```python
from build123d import *

# Parameters (mm, degrees)
SKICA1_R                  = 30
SKICA1_R_2                = 15
P_IDAT_VYSUNUT_M1_DEPTH   = 80
ZKOSEN_1_SIZE             = 1
M8_Z_VIT1_REACH           = 62
M8_Z_VIT1_BORE_R          = 3.4
M8_Z_VIT1_ON_FACE_2_REACH = 72.981
M8_Z_VIT1_BORE_2_R        = 3.4
M8_Z_VIT2_REACH           = 62
M8_Z_VIT2_BORE_R          = 3.4
KRUHOV_POLE1_COUNT        = 2
KRUHOV_POLE1_ANGLE        = 30


with BuildPart() as part:
    # Skica1 → Přidat vysunutím1 (new body)
    with BuildSketch(Plane.XY):
        Circle(SKICA1_R)
        Circle(SKICA1_R_2, mode=Mode.SUBTRACT)
    extrude(amount=P_IDAT_VYSUNUT_M1_DEPTH)

    # Zkosení1
    zkosen_1_edges = [part.edges().sort_by_distance(p)[0] for p in [
        (-30, 0, 0),
        (-30, 0, 80),
        (-15, 0, 0),
        (-15, 0, 80),
    ]]
    chamfer(zkosen_1_edges, length=ZKOSEN_1_SIZE)

    # M8 závit1 bore (on position points) → M8 závit1 (cut, up to next)
    with BuildSketch(Plane(origin=(0, -30, 20), x_dir=(-1, 0, 0), z_dir=(0, -1, 0)), mode=Mode.PRIVATE) as m8_z_vit1_sk1:
        Circle(M8_Z_VIT1_BORE_R)
    m8_z_vit1_tool1 = extrude(m8_z_vit1_sk1.sketch, amount=-M8_Z_VIT1_REACH, mode=Mode.PRIVATE) & part.part
    add(m8_z_vit1_tool1.solids().sort_by_distance((0, -30, 20))[0], mode=Mode.SUBTRACT)

    # M8 závit1 bore 2 (on position points) → M8 závit1 on face 2 (cut, up to next)
    with BuildSketch(Plane(origin=(15, -25.980762114, 20), x_dir=(-0.866025303, -0.500000175, 0), z_dir=(0.500000175, -0.866025303, 0)), mode=Mode.PRIVATE) as m8_z_vit1_on_face_2_sk1:
        Circle(M8_Z_VIT1_BORE_2_R)
    m8_z_vit1_on_face_2_tool1 = extrude(m8_z_vit1_on_face_2_sk1.sketch, amount=-M8_Z_VIT1_ON_FACE_2_REACH, mode=Mode.PRIVATE) & part.part
    add(m8_z_vit1_on_face_2_tool1.solids().sort_by_distance((15, -25.980762, 20))[0], mode=Mode.SUBTRACT)

    # M8 závit2 bore → M8 závit2 (cut, up to next)
    with BuildSketch(Plane(origin=(30, 0, 0), x_dir=(0, 0, -1), z_dir=(1, 0, 0)), mode=Mode.PRIVATE) as m8_z_vit2_sk1:
        with Locations((-60, 0)):
            Circle(M8_Z_VIT2_BORE_R)
    m8_z_vit2_tool1 = extrude(m8_z_vit2_sk1.sketch, amount=-M8_Z_VIT2_REACH, mode=Mode.PRIVATE) & part.part
    m8_z_vit2 = m8_z_vit2_tool1.solids().sort_by_distance((30, 0, 60))[0]
    add(m8_z_vit2, mode=Mode.SUBTRACT)

    # Kruhové pole1: M8 závit2 ×2 about axis
    kruhov_pole1_axis = Axis((0, 0, 80), (0, 0, 1))
    for i in range(1, KRUHOV_POLE1_COUNT):
        add(m8_z_vit2.rotate(kruhov_pole1_axis, i * KRUHOV_POLE1_ANGLE / (KRUHOV_POLE1_COUNT - 1)), mode=Mode.SUBTRACT)


solid = part.part
```
Can you work these out from the model? Positions are in its coordinate system, mm. Give positions to 0.01 mm unless a question says otherwise; leave off trailing zeros. Loops run counter-clockwise (first coordinate to the right, second up) from the corner with the lowest first, then second, coordinate; pieces in that order, holes last. Notation, with made-up numbers: M 60.25,4.25 L 101.25,4.25 A12 cw 101.25,22.25 Z; hole C 30,24 d11. An arc over 180 degrees is marked long. Use CSV: the item, a comma, the result in double quotes. Start each with the question number.
1. Imagine slicing it at B-B, the plane y = 0. Write out the boundary of the cut face in (x, z), plus the area to 3 significant figures.
2. Imagine slicing it at C-C, the plane z = 20. Write out the boundary of the cut face in (x, y).
3. Imagine slicing it at A-A, the plane x = 0. Write out the boundary of the cut face in (y, z), plus the area to 3 significant figures.
4. If we mould it in two halves opening along Y, with no side actions, what happens to faces 1 (the face through (0.74, -22.41, 23.32)), 2 (the face through (9.85, -20.19, 23.02)), 3 (the face through (22.41, -1.3, 56.86)), 4 (the face through (-22.111, 20.275, 39.454))? For each: released by +Y, released by -Y, zero draft, split by the parting line, or undercut.
5. For P1, Ø1.5, axis at x = -8, z = 16.5, coming from the +Y side; P2, Ø9, axis at x = 0, z = 20, coming from the +Y side; P3, Ø4, axis at y = 18, z = 40.5, coming from the -X side, each with a flat end and sliding along its axis, tell me the tip position at first contact or that it passes through.
6. Imagine slicing it at D-D, the plane z = 74. Write out the boundary of the cut face in (x, y), plus the area to 3 significant figures.
7. If I drill on L1, parallel to Z at x = 0, y = -17.75; L2, parallel to X at y = -24, z = 20; L3, parallel to Z at x = 22, y = 0, over which ranges is the centre line in solid material (lowest first)?
Response values:
1,outline,"M -30,1 L -29,0 L -16,0 L -15,1 L -15,79 L -16,80 L -29,80 L -30,79 Z; M 15,1 L 16,0 L 29,0 L 30,1 L 30,56.6 L 15,56.6 Z; M 15,63.4 L 30,63.4 L 30,79 L 29,80 L 16,80 L 15,79 Z"
1,area,"2,290 mm^2"
2,outline,"M -3.4,-29.81 L -3.4,-14.61 A15 cw long 10.25,-10.95 L 17.85,-24.11 A30 ccw long Z; M 3.4,-29.81 A30 ccw 11.96,-27.51 L 4.36,-14.35 A15 cw 3.4,-14.61 Z"
3,outline,"M -30,1 L -29,0 L -16,0 L -15,1 L -15,16.6 L -30,16.6 Z; M -30,23.4 L -15,23.4 L -15,79 L -16,80 L -29,80 L -30,79 Z; M 15,1 L 16,0 L 29,0 L 30,1 L 30,79 L 29,80 L 16,80 L 15,79 Z"
3,area,"2,290 mm^2"
4,face 1,"zero draft"
4,face 2,"undercut"
4,face 3,"undercut"
4,face 4,"split by the parting line"
5,P1,"y = 29.11"
5,P2,"y = 30"
5,P3,"x = -25.38"
6,outline,"C 0,0 d60; hole C 0,0 d30"
6,area,"2,120 mm^2"
7,L1,"0 to 16.6, 23.4 to 80"
7,L2,"-18 to -3.4, 3.4 to 9.93, 17.78 to 18"
7,L3,"0 to 56.6, 63.4 to 80"
